Check sheet for the modelled part. Datum: model origin and axes. Units: mm. Round coordinates to 2 decimals unless told otherwise and drop trailing zeros. Order: outer loops, then holes, each group sorted by start corner. A loop starts at its lowest first (then second) coordinate and runs counter-clockwise, first axis right, second up.
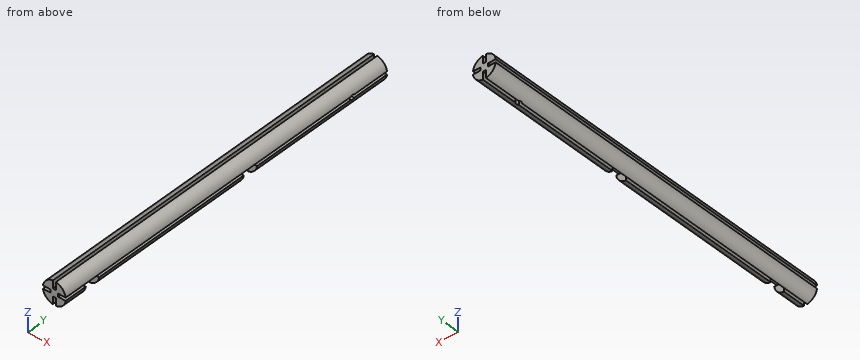
```python
from build123d import *

# Parameters (mm, degrees)
BOSS_EXTRUDE2_DEPTH     = 4000
CUT_EXTRUDE1_START      = 200
SKETCH2_W               = 74.330343737
SKETCH2_H               = 74.330343737
CUT_EXTRUDE1_DEPTH      = 50
CUT_EXTRUDE2_START      = 1380
SKETCH2_2_W             = 74.330343737
SKETCH2_2_H             = 74.330343737
CUT_EXTRUDE2_DEPTH      = 50
SKETCH3_R               = 15.2
CUT_EXTRUDE3_DEPTH      = 49.330343737
SKETCH4_R               = 15.2
CUT_EXTRUDE4_DEPTH      = 49.330343737
CUT_EXTRUDE5_DEPTH      = 4002.923477282
CUT_EXTRUDE5_DEPTH_BACK = 4002.923477282
SKETCH5_W               = 148.660687474
SKETCH5_H               = 1600


with BuildPart() as part:
    # Sketch1 → Boss-Extrude2 (new body)
    with BuildSketch(Plane(origin=(0, 0, 0), x_dir=(1, 0, 0), z_dir=(0, 1, 0))):
        with BuildLine():
            Line((-10, 74.330343737), (-10, 25))
            Line((-10, 25), (10, 25))
            Line((10, 25), (10, 74.330343737))
            ThreePointArc((10, 74.330343737), (53.033008589, 53.033008589), (74.330343737, 10))
            Line((74.330343737, 10), (25, 10))
            Line((25, 10), (25, -10))
            Line((25, -10), (74.330343737, -10))
            ThreePointArc((74.330343737, -10), (53.033008589, -53.033008589), (10, -74.330343737))
            Line((10, -74.330343737), (10, -25))
            Line((10, -25), (-10, -25))
            Line((-10, -25), (-10, -74.330343737))
            ThreePointArc((-10, -74.330343737), (-53.033008589, -53.033008589), (-74.330343737, -10))
            Line((-74.330343737, -10), (-25, -10))
            Line((-25, -10), (-25, 10))
            Line((-25, 10), (-74.330343737, 10))
            ThreePointArc((-74.330343737, 10), (-53.033008589, 53.033008589), (-10, 74.330343737))
        make_face()
    extrude(amount=BOSS_EXTRUDE2_DEPTH)

    # Sketch2 → Cut-Extrude1 (cut, symmetric)
    with BuildSketch(Plane(origin=(0, 0, 0), x_dir=(1, 0, 0), z_dir=(0, 1, 0)).offset(CUT_EXTRUDE1_START)):
        with Locations((37.165171869, 37.165171869)):
            Rectangle(SKETCH2_W, SKETCH2_H)
    extrude(amount=CUT_EXTRUDE1_DEPTH, both=True, mode=Mode.SUBTRACT)

    # Sketch2<2> → Cut-Extrude2 (cut, symmetric)
    with BuildSketch(Plane(origin=(0, 0, 0), x_dir=(1, 0, 0), z_dir=(0, 1, 0)).offset(CUT_EXTRUDE2_START)):
        with Locations((37.165171869, 37.165171869)):
            Rectangle(SKETCH2_2_W, SKETCH2_2_H)
    extrude(amount=CUT_EXTRUDE2_DEPTH, both=True, mode=Mode.SUBTRACT)

    # Sketch3 → Cut-Extrude3 (cut)
    with BuildSketch(Plane(origin=(74.330343737, 0, 0), x_dir=(0, 0, -1), z_dir=(1, 0, 0))):
        with Locations((0, 2143)):
            Circle(SKETCH3_R)
    extrude(amount=-CUT_EXTRUDE3_DEPTH, mode=Mode.SUBTRACT)

    # Sketch4 → Cut-Extrude4 (cut)
    with BuildSketch(Plane(origin=(0, 0, -74.330343737), x_dir=(-1, 0, 0), z_dir=(0, 0, -1))):
        with Locations((0, 2143)):
            Circle(SKETCH4_R)
    extrude(amount=-CUT_EXTRUDE4_DEPTH, mode=Mode.SUBTRACT)

    # Sketch5 → Cut-Extrude5 (cut, two sides: drawn at the far end of the back side and taken through both)
    with BuildSketch(Plane.XY.offset(25).offset(-CUT_EXTRUDE5_DEPTH_BACK)):
        with Locations((0, 3200)):
            Rectangle(SKETCH5_W, SKETCH5_H)
    extrude(amount=CUT_EXTRUDE5_DEPTH + CUT_EXTRUDE5_DEPTH_BACK, mode=Mode.SUBTRACT)


solid = part.part
```
Item 1: Scan lines: line 1 along Y through (x, z) = (51.5, -42.5); line 2 along Z through (x, y) = (-12, 836.5); line 3 along Z through (x, y) = (2, 921.5). Record each from-to range of solid material in increasing order.
Answer:
line 1: y = 0 to 150, 250 to 1330, 1430 to 2400
line 2: z = -74.03 to 74.03
line 3: z = -25 to 25
Item 2: Sectioned sample at A-A (y = 2219). Record the cut outline in (x, z), and give its area (3 significant figures).
Answer:
outline: (-74.33, -10) arc R75 ccw to (-10, -74.33) - (-10, -25) - (10, -25) - (10, -74.33) arc R75 ccw to (74.33, -10) - (25, -10) - (25, 10) - (74.33, 10) arc R75 ccw to (10, 74.33) - (10, 25) - (-10, 25) - (-10, 74.33) arc R75 ccw to (-74.33, 10) - (-25, 10) - (-25, -10) - close
area: 13,700 mm2
Item 3: Go/stop test with flat-tipped pins: P1, Ø24.5, axis at x = -43, y = 885, coming from the +Z side; P2, Ø5, axis at y = 966, z = 59.5, coming from the +X side; P3, Ø6, axis at x = 2.5, y = 730, coming from the +Z side. Record where each tip stops, or that it passes through.
Answer:
P1: stops at z = 68.41
P2: stops at x = 48.74
P3: stops at z = 25
